Work out the finished part from the listing and answer in its coordinate system (mm). A direction names the side the tool comes from. Round coordinates to 2 decimals unless told otherwise and drop trailing zeros. Order: outer loops, then holes, each group sorted by start corner. A loop starts at its lowest first (then second) coordinate and runs counter-clockwise, first axis right, second up. Notation, with made-up numbers: (10, 58) - (53, 58) arc R19 ccw to (53, 68) - close; hole circle Ø1 at (16.25, 54.25). An arc over 180 degrees is marked (long way). Answer in a Markdown table with one row per item.
from build123d import *

# Parameters (mm, degrees)
BOSS_EXTRUDE1_DEPTH     = 3.81
SKETCH2_R               = 2.38125
CUT_EXTRUDE1_DEPTH      = 8.62
CHAMFER1_SIZE           = 0.508
CHAMFER1_SIZE2          = 1.66159313
CHAMFER2_SIZE           = 0.508
CHAMFER2_SIZE2          = 1.66159313
CHAMFER3_SIZE           = 0.508
CHAMFER3_SIZE2          = 1.66159313
CHAMFER4_SIZE           = 0.508
CHAMFER4_SIZE2          = 1.66159313
SKETCH3_R               = 1.5875
CUT_EXTRUDE2_DEPTH      = 12.7
CHAMFER5_SIZE           = 0.508
CHAMFER5_SIZE2          = 1.66159313
CHAMFER5_PART_2_SIZE    = 0.508
CHAMFER5_PART_2_SIZE2   = 1.66159313
SKETCH4_R               = 4.826
CUT_EXTRUDE3_DEPTH      = 8.62
FILLET1_R               = 2.54
SKETCH5_R               = 1.830021078
SKETCH5_R_2             = 1.859210554
CUT_EXTRUDE4_DEPTH      = 12.7
CHAMFER6_SIZE           = 0.508
CHAMFER6_SIZE2          = 1.66159313
CHAMFER6_PART_2_SIZE    = 0.508
CHAMFER6_PART_2_SIZE2   = 1.66159313
CUT_EXTRUDE7_START      = 10.16
CUT_EXTRUDE7_DEPTH      = 42.745681687
CUT_EXTRUDE7_DEPTH_BACK = 6.35


with BuildPart() as part:
    # Sketch1 → Boss-Extrude1 (new body, symmetric)
    with BuildSketch(Plane(origin=(0, 0, 0), x_dir=(0, 0, -1), z_dir=(1, 0, 0))):
        with BuildLine():
            Line((-5.401607261, 20.422717891), (-10.431909051, 20.422717891))
            ThreePointArc((-10.431909051, 20.422717891), (-11.089309426, 20.33616949), (-11.701909051, 20.082422416))
            Line((-11.701909051, 20.082422416), (-40.393951745, 3.517063844))
            ThreePointArc((-40.393951745, 3.517063844), (-41.32365627, 2.587359318), (-41.663951745, 1.317359318))
            Line((-41.663951745, 1.317359318), (-41.663951745, -8.787282109))
            ThreePointArc((-41.663951745, -8.787282109), (-40.920002969, -10.583333333), (-39.123951745, -11.327282109))
            Line((-39.123951745, -11.327282109), (19.155833333, -11.327282109))
            ThreePointArc((19.155833333, -11.327282109), (20.951884558, -10.583333333), (21.695833333, -8.787282109))
            Line((21.695833333, -8.787282109), (21.695833333, 8.787282109))
            ThreePointArc((21.695833333, 8.787282109), (21.502487346, 9.759298027), (20.951884558, 10.583333333))
            Line((20.951884558, 10.583333333), (11.856448776, 19.678769115))
            ThreePointArc((11.856448776, 19.678769115), (11.03241347, 20.229371903), (10.060397552, 20.422717891))
            Line((10.060397552, 20.422717891), (5.401607261, 20.422717891))
            ThreePointArc((5.401607261, 20.422717891), (4.040314071, 20.027124767), (3.10305098, 18.963568955))
            ThreePointArc((3.10305098, 18.963568955), (0, 16.993717891), (-3.10305098, 18.963568955))
            ThreePointArc((-3.10305098, 18.963568955), (-4.040314071, 20.027124767), (-5.401607261, 20.422717891))
        make_face()
    extrude(amount=BOSS_EXTRUDE1_DEPTH, both=True)

    # Sketch2 → Cut-Extrude1 (cut, through all)
    with BuildSketch(Plane(origin=(3.81, 0, 0), x_dir=(0, 0, -1), z_dir=(1, 0, 0))):
        with Locations((14.552083333, 6.275759092)):
            Circle(SKETCH2_R)
        with Locations((0, 2.376540114)):
            Circle(SKETCH2_R)
        with Locations((-20.497285078, -3.115690869)):
            Circle(SKETCH2_R)
    extrude(amount=-CUT_EXTRUDE1_DEPTH, mode=Mode.SUBTRACT)

    # Chamfer1
    chamfer1_edges = [part.edges().sort_by_distance(p)[0] for p in [
        (3.81, 6.275759092, -12.170833333),
        (3.81, 2.376540114, 2.38125),
        (3.81, -3.115690869, 22.878535078),
    ]]
    chamfer1_side = [part.faces().sort_by_distance(p)[0] for p in [
        (3.81, 2.381626515, 7.750929536),
    ]]
    chamfer(chamfer1_edges, length=CHAMFER1_SIZE, length2=CHAMFER1_SIZE2, reference=chamfer1_side[0])

    # Chamfer2
    chamfer2_edges = [part.edges().sort_by_distance(p)[0] for p in [
        (-3.81, -3.115690869, 22.878535078),
    ]]
    chamfer2_side = [part.faces().sort_by_distance(p)[0] for p in [
        (-3.81, 2.381626515, 7.750929536),
    ]]
    chamfer(chamfer2_edges, length=CHAMFER2_SIZE, length2=CHAMFER2_SIZE2, reference=chamfer2_side[0])

    # Chamfer3
    chamfer3_edges = [part.edges().sort_by_distance(p)[0] for p in [
        (-3.81, 2.376540114, 2.38125),
    ]]
    chamfer3_side = [part.faces().sort_by_distance(p)[0] for p in [
        (-3.81, 2.410504504, 7.683971585),
    ]]
    chamfer(chamfer3_edges, length=CHAMFER3_SIZE, length2=CHAMFER3_SIZE2, reference=chamfer3_side[0])

    # Chamfer4
    chamfer4_edges = [part.edges().sort_by_distance(p)[0] for p in [
        (-3.81, 6.275759092, -12.170833333),
    ]]
    chamfer4_side = [part.faces().sort_by_distance(p)[0] for p in [
        (-3.81, 2.410683864, 7.724549459),
    ]]
    chamfer(chamfer4_edges, length=CHAMFER4_SIZE, length2=CHAMFER4_SIZE2, reference=chamfer4_side[0])

    # Sketch3 → Cut-Extrude2 (cut)
    with BuildSketch(Plane(origin=(0, 20.422717891, 0), x_dir=(1, 0, 0), z_dir=(0, 1, 0))):
        with Locations((0, -7.916758156)):
            Circle(SKETCH3_R)
        with Locations((0, 7.731002406)):
            Circle(SKETCH3_R)
    extrude(amount=-CUT_EXTRUDE2_DEPTH, mode=Mode.SUBTRACT)

    # Chamfer5
    chamfer5_edges = [part.edges().sort_by_distance(p)[0] for p in [
        (-1.5875, 20.422717891, 7.916758156),
    ]]
    chamfer5_side = [part.faces().sort_by_distance(p)[0] for p in [
        (0, 20.422717891, 5.492913524),
    ]]
    chamfer(chamfer5_edges, length=CHAMFER5_SIZE, length2=CHAMFER5_SIZE2, reference=chamfer5_side[0])

    # Chamfer5 part 2
    chamfer5_part_2_edges = [part.edges().sort_by_distance(p)[0] for p in [
        (-1.5875, 20.422717891, -7.731002406),
    ]]
    chamfer5_part_2_side = [part.faces().sort_by_distance(p)[0] for p in [
        (0, 20.422717891, -9.971084212),
    ]]
    chamfer(chamfer5_part_2_edges, length=CHAMFER5_PART_2_SIZE, length2=CHAMFER5_PART_2_SIZE2, reference=chamfer5_part_2_side[0])

    # Sketch4 → Cut-Extrude3 (cut, through all)
    with BuildSketch(Plane.ZY.offset(3.81)):
        with Locations((0, -11.327282109)):
            Circle(SKETCH4_R)
    extrude(amount=-CUT_EXTRUDE3_DEPTH, mode=Mode.SUBTRACT)

    # Fillet1
    fillet1_edges = [part.edges().sort_by_distance(p)[0] for p in [
        (0, -11.327282109, -4.826),
        (0, -11.327282109, 4.826),
    ]]
    fillet(fillet1_edges, radius=FILLET1_R)

    # Sketch5 → Cut-Extrude4 (cut)
    with BuildSketch(Plane.XZ.offset(11.327282109)):
        with Locations((0, -13.035023694)):
            Circle(SKETCH5_R)
        with Locations((0, 13.035023694)):
            Circle(SKETCH5_R_2)
    extrude(amount=-CUT_EXTRUDE4_DEPTH, mode=Mode.SUBTRACT)

    # Chamfer6
    chamfer6_edges = [part.edges().sort_by_distance(p)[0] for p in [
        (-1.830021078, -11.327282109, -13.035023694),
    ]]
    chamfer6_side = [part.faces().sort_by_distance(p)[0] for p in [
        (3.665805117, -11.327282109, -13.035023694),
    ]]
    chamfer(chamfer6_edges, length=CHAMFER6_SIZE, length2=CHAMFER6_SIZE2, reference=chamfer6_side[0])

    # Chamfer6 part 2
    chamfer6_part_2_edges = [part.edges().sort_by_distance(p)[0] for p in [
        (-1.859210554, -11.327282109, 13.035023694),
    ]]
    chamfer6_part_2_side = [part.faces().sort_by_distance(p)[0] for p in [
        (0, -11.327282109, 23.481278136),
    ]]
    chamfer(chamfer6_part_2_edges, length=CHAMFER6_PART_2_SIZE, length2=CHAMFER6_PART_2_SIZE2, reference=chamfer6_part_2_side[0])

    # Sketch7 → Cut-Extrude7 (cut, two sides)
    with BuildSketch(Plane(origin=(0, 0, 0), x_dir=(1, 0, 0), z_dir=(0, -0.5, 0.866025404)).offset(CUT_EXTRUDE7_START)) as cut_extrude7_sk:
        Polygon((-10.16, 27.687842508), (10.16, 27.687842508), (10.16, 14.987842508), (0, 25.147842508), (-10.16, 14.987842508), align=None)
    extrude(amount=CUT_EXTRUDE7_DEPTH, mode=Mode.SUBTRACT)
    extrude(cut_extrude7_sk.sketch, amount=-CUT_EXTRUDE7_DEPTH_BACK, mode=Mode.SUBTRACT)


solid = part.part
1) Each of these flat-tipped pins is pushed along its axis until it touches: pin 1 (7.5 mm diameter, centred on y = -3.12, z = 20.5, fed in from +X); pin 2 (1.1 mm diameter, centred on x = -0.5, z = 12.5, fed in from -Y); pin 3 (1 mm diameter, centred on x = 0.5, z = 8.5, fed in from +Y); pin 4 (3 mm diameter, centred on x = 0, z = 13.04, fed in from +Y). Where does it stop, or does it pass through?
Filled in:
| item | result |
|---|---|
| pin 1 | stops at x = 3.81 |
| pin 2 | stops at y = 1.37 |
| pin 3 | stops at y = 7.72 |
| pin 4 | stops at y = 20.17 |
2) The mould has two halves that part along X. Classify faces 4 (the face through (-1.37, -4.22, 14.29)), 5 (the face through (-0.05, -6.5, 0.08)), 6 (the face through (0, 7.723, 8)), 7 (the face through (-2.84, 9.53, 28.11)): released by +X, released by -X, zero draft, split by the parting line, or undercut.
Filled in:
| item | result |
|---|---|
| face 4 | undercut |
| face 5 | zero draft |
| face 6 | undercut |
| face 7 | released by -X |
3) Find section B-B, the plane y = 16. Give the vertices of the cut face in (x, z) (1 decimal).
Filled in:
| item | result |
|---|---|
| outline | (-3.8, -15.5) - (3.8, -15.5) - (3.8, 15) - (1.9, 18.8) - (-1.9, 18.8) - (-3.8, 15) - close; hole circle Ø3.2 at (0, -7.7); hole circle Ø3.2 at (0, 7.9) |
4) Find section C-C, the plane x = 0.5. Give the number of separate pieces and of enclosed holes in the cut face, then the cut area to 3 significant figures.
Filled in:
| item | result |
|---|---|
| separate pieces | 1 |
| enclosed holes | 3 |
| area | 1,400 mm^2 |
5) Find the intervals of material crossed by probe 1 along Z at (x, y) = (0.75, -8); probe 2 along Z at (x, y) = (0.75, 16); probe 3 along Z at (x, y) = (-1.25, -6), in increasing order. Write a range as from..to.
Filled in:
| item | result |
|---|---|
| probe 1 | z = -21.7..-14.7, -11.37..-3.5, 3.5..11.33, 14.74..41.66 |
| probe 2 | z = -15.54..-9.13, -6.33..6.52, 9.32..18.77 |
| probe 3 | z = -21.7..-14.37, -11.7..11.66, 14.41..41.66 |
6) Find section A-A, the plane z = 0. Give the vertices of the cut face in (x, y), then the cut area to 3 significant figures.
Filled in:
| item | result |
|---|---|
| outline | (-3.81, -6.5) - (3.81, -6.5) - (3.81, -0.51) - (2.15, 0) - (-2.15, 0) - (-3.81, -0.51) - close; (-3.81, 5.27) - (-2.15, 4.76) - (2.15, 4.76) - (3.81, 5.27) - (3.81, 16.99) - (-3.81, 16.99) - close |
| area | 141 mm^2 |
7) Find section D-D, the plane z = 29. Give the vertices of the cut face in (x, y) (3 decimals).
Filled in:
| item | result |
|---|---|
| outline | (-3.81, -11.327) - (3.81, -11.327) - (3.81, 7.896) - (1.905, 10.095) - (-1.905, 10.095) - (-3.81, 7.896) - close |
8) Which of the six approach directions +Z, -Z, +X, -X, +Y, -Y give full straight-line access (tool end or side, diameter ignored) to faces 1 (the face through (-3.267, 17.777, 14.663)), 2 (the face through (0.733, 13.319, 9.325)), 3 (the face through (0, 20, -4))?
Filled in:
| item | result |
|---|---|
| face 1 | +Z, -X |
| face 2 | +Y |
| face 3 | +X, -X, +Y |
